```python
from build123d import *

# Parameters (mm, degrees)
F2_R = 1.19999
F3_R = 1.5


# Not quite as in the source:
# - a fillet or chamfer is up to 0.001 mm smaller than in the source, because OpenCascade refuses the exact size


with BuildPart() as f1:
    # F0 (on Front) → F1 (revolve)
    with BuildSketch(Plane.XZ):
        with BuildLine():
            Line((0, 22.8), (0, 24))
            ThreePointArc((0, 24), (-13.8564064606, 16), (-13.8564064606, 0))
            Line((-13.8564064606, 0), (-12.451505933, 0))
            ThreePointArc((-12.451505933, 0), (-13.8029789452, 13.3402033893), (-3.825, 22.2971806661))
            ThreePointArc((-3.825, 22.2971806661), (-3.227786159, 22.4437320839), (-2.625, 22.5653484339))
            ThreePointArc((-2.625, 22.5653484339), (-1.3177335047, 22.741220384), (0, 22.8))
        make_face()
        with BuildLine():
            Line((-2.625, 18.0653484339), (-2.625, 22.5653484339))
            ThreePointArc((-2.625, 22.5653484339), (-3.227786159, 22.4437320839), (-3.825, 22.2971806661))
            Line((-3.825, 22.2971806661), (-3.825, 18.0653484339))
            Line((-3.825, 18.0653484339), (-2.625, 18.0653484339))
        make_face()
    revolve(axis=Axis((0, 0, 23.4), (0, 0, 1)))

    # F2 (radius 1.2 in the source; OpenCascade refuses exactly that, so slightly less here)
    f2_edges = [f1.edges().sort_by_distance(p)[0] for p in [
        (2.625, 0, 18.065348),
    ]]
    fillet(f2_edges, radius=F2_R)

    # F3
    f3_edges = [f1.edges().sort_by_distance(p)[0] for p in [
        (3.825, 0, 22.297181),
    ]]
    fillet(f3_edges, radius=F3_R)


solid = f1.part
```
Input: part model. Units: mm. Frame: model coordinates. Give positions to 0.01 mm unless a question says otherwise; leave off trailing zeros. Order: outer loops, then holes, each group sorted by start corner. A loop starts at its lowest first (then second) coordinate and runs counter-clockwise, first axis right, second up.
1. Section A-A on x = 7.5. Return the cut outline in (y, z).
Derived:
outline: (-11.65, 0) - (-9.94, 0) arc R12.76 cw (long way) to (9.94, 0) - (11.65, 0) arc R14.13 ccw (long way) to start
2. Section C-C on z = 15.75. Return the cut outline in (x, y), and give its area (3 significant figures).
Derived:
outline: circle Ø28 at (0, 0); hole circle Ø25.22 at (0, 0)
area: 116 mm2
3. Section B-B on y = -11.5. Return the cut outline in (x, z), and give its area (3 significant figures).
Derived:
outline: (-7.73, 0) - (-4.77, 0) arc R9.32 cw (long way) to (4.77, 0) - (7.73, 0) arc R11.12 ccw (long way) to start
area: 91.4 mm2
4. Material intervals for L1, parallel to Y at x = 0, z = 20.6 (3 decimals); L2, parallel to X at y = 0, z = 21.35 (3 decimals); L3, parallel to X at y = 0, z = 20.5 (1 decimal), sorted ascending.
Derived:
L1: y = -9.861 to -7.764, -3.883 to -2.625, 2.625 to 3.883, 7.764 to 9.861
L2: x = -8.819 to -6.389, -4.377 to -2.625, 2.625 to 4.377, 6.389 to 8.819
L3: x = -10 to -7.9, -3.9 to -2.6, 2.6 to 3.9, 7.9 to 10
5. Pin query (flat end, axial travel): pin 1 (6 mm diameter, centred on y = -0.5, z = 17, fed in from -X); pin 2 (10 mm diameter, centred on x = -11, z = 8.5, fed in from +Y); pin 3 (2.5 mm diameter, centred on x = -1, y = 0.5, fed in from -Z). Return the tip coordinate at first contact, or that it passes through.
Derived:
pin 1: stops at x = -14.83
pin 2: stops at y = 14.83
pin 3: stops at z = 22.61
